from build123d import *

# Parameters (mm, degrees)
SKETCH_1_W          = 78
SKETCH_1_H          = 52
EXTRUDE_1_DEPTH     = 3
SKETCH_2_R          = 1.6
CUT_EXTRUDE_1_DEPTH = 3
SKETCH_7_R          = 1.6
CUT_EXTRUDE_2_DEPTH = 3
FILLET_1_R          = 3


with BuildPart() as part:
    # 草图1 → 凸台-拉伸1 (new body)
    with BuildSketch(Plane(origin=(0, 0, 0), x_dir=(1, 0, 0), z_dir=(0, 1, 0))):
        Rectangle(SKETCH_1_W, SKETCH_1_H)
    extrude(amount=EXTRUDE_1_DEPTH)

    # 草图2 → 切除-拉伸1 (cut)
    with BuildSketch(Plane(origin=(0, 3, 0), x_dir=(1, 0, 0), z_dir=(0, 1, 0))):
        with BuildLine():
            ThreePointArc((-32.8, 21.4), (-33.26862915, 22.53137085), (-34.4, 23))
            Line((-34.4, 23), (-34.4, 21.4))
            Line((-34.4, 21.4), (-36, 21.4))
            ThreePointArc((-36, 21.4), (-34.4, 19.8), (-32.8, 21.4))
        make_face()
        with BuildLine():
            Line((-34.4, 21.4), (-34.4, 23))
            ThreePointArc((-34.4, 23), (-35.53137085, 22.53137085), (-36, 21.4))
            Line((-36, 21.4), (-34.4, 21.4))
        make_face()
        with BuildLine():
            ThreePointArc((36, 21.4), (35.53137085, 22.53137085), (34.4, 23))
            Line((34.4, 23), (34.4, 21.4))
            Line((34.4, 21.4), (36, 21.4))
        make_face()
        with BuildLine():
            Line((34.4, 21.4), (34.4, 23))
            ThreePointArc((34.4, 23), (33.26862915, 20.26862915), (36, 21.4))
            Line((36, 21.4), (34.4, 21.4))
        make_face()
        with BuildLine():
            ThreePointArc((36, -21.4), (33.26862915, -20.26862915), (34.4, -23))
            Line((34.4, -23), (34.4, -21.4))
            Line((34.4, -21.4), (36, -21.4))
        make_face()
        with BuildLine():
            Line((34.4, -21.4), (34.4, -23))
            ThreePointArc((34.4, -23), (35.53137085, -22.53137085), (36, -21.4))
            Line((36, -21.4), (34.4, -21.4))
        make_face()
        with Locations(Location((-34.4, -21.4, 0), (0, 0, 270))):
            Circle(SKETCH_2_R)
    extrude(amount=-CUT_EXTRUDE_1_DEPTH, mode=Mode.SUBTRACT)

    # 草图7 → 切除-拉伸2 (cut)
    with BuildSketch(Plane(origin=(0, 3, 0), x_dir=(1, 0, 0), z_dir=(0, 1, 0))):
        with Locations(Location((-30, -9, 0), (0, 0, 270))):
            Circle(SKETCH_7_R)
        with Locations(Location((-27, 9, 0), (0, 0, 270))):
            Circle(SKETCH_7_R)
        with Locations(Location((27, 9, 0), (0, 0, 270))):
            Circle(SKETCH_7_R)
        with Locations(Location((30, -9, 0), (0, 0, 270))):
            Circle(SKETCH_7_R)
    extrude(amount=-CUT_EXTRUDE_2_DEPTH, mode=Mode.SUBTRACT)

    # 圆角1
    fillet_1_edges = [part.edges().sort_by_distance(p)[0] for p in [
        (39, 1.5, 26),
        (-39, 1.5, 26),
        (-39, 1.5, -26),
        (39, 1.5, -26),
    ]]
    fillet(fillet_1_edges, radius=FILLET_1_R)


solid = part.part
Check sheet for the modelled part. Datum: model origin and axes. Units: mm. Coordinates: 2 decimals unless noted, no trailing zeros. Write each loop counter-clockwise with the first axis right and the second up, starting at its lowest first coordinate (ties: lowest second). Pieces come first, ordered by that corner, then holes.
Item 1: Scan lines: probe 1 along X at (y, z) = (2.6, 21.5); probe 2 along X at (y, z) = (1.85, -9); probe 3 along Z at (x, y) = (34.4, 1). Record each from-to range of solid material in increasing order.
Numbers:
probe 1: x = -39 to -36, -32.8 to 32.8, 36 to 39
probe 2: x = -39 to -28.6, -25.4 to 25.4, 28.6 to 39
probe 3: z = -26 to -23, -19.8 to 19.8, 23 to 26
Item 2: Mould release check, pull along Z, two halves, no side actions. Record for faces 1 (the face through (-39, 1, 0)), 2 (the face through (-28.414, 1.521, 8.792)), 3 (the face through (-33.05, 1.52, 22.26)), 4 (the face through (-38.14, 1.52, -25.1)): released by +Z, released by -Z, zero draft, split by the parting line, or undercut.
Numbers:
face 1: zero draft
face 2: undercut
face 3: undercut
face 4: released by -Z
Item 3: Cross-section at A-A on x = -27. Record the boundary of the cut face in (y, z), then the cut area to 3 significant figures.
Numbers:
outline: (0, -26) - (3, -26) - (3, -10.6) - (0, -10.6) - close; (0, -7.4) - (3, -7.4) - (3, 26) - (0, 26) - close
area: 146 mm2
Item 4: Depth check by flat-ended pin: pin 1 Ø3.5 at (x, z) = (34.4, -21.4) entering from +Y. Enter the tip coordinate at first touch or a pass-through.
Numbers:
pin 1: stops at y = 3
Item 5: Cross-section at B-B on y = 1.6. Count the separate pieces of the cut face and the enclosed holes in it, then the cut area to 3 significant figures.
Numbers:
separate pieces: 1
enclosed holes: 8
area: 3,980 mm2
